For this review, take the finished solid that the model builds, in its own axes (mm). A direction names the side the tool comes from. Round coordinates to 2 decimals unless told otherwise and drop trailing zeros. Order: outer loops, then holes, each group sorted by start corner. A loop starts at its lowest first (then second) coordinate and runs counter-clockwise, first axis right, second up. Notation, with made-up numbers: (41.5, 38) -> (97.5, 38) arc R20 cw to (97.5, 54) -> close; hole circle Ø10 at (33.5, 9). An arc over 180 degrees is marked (long way). Use a Markdown table: item, result. Add a question column.
1) Machinability: for faces 1 (the face through (0.176, 5.803, -7.998)), 2 (the face through (6.05, 3, 6)), 3 (the face through (9.82, 2.96, 4.94)), which of the approach directions +Z, -Z, +X, -X, +Y, -Y give a long, thin tool a straight path to every point of the face, cutting with its end or side? Answer none if there is none.
2) Consider section C-C (y = 5.1). State the section outline as (x, z) points, plus the area to 3 significant figures.
3) Consider section A-A (x = 0). State the section outline as (y, z) points, plus the area to 3 significant figures.
4) Consider section B-B (z = -1.75). State the section outline as (x, y) points.
5) Consider section D-D (z = 9.5). State the section outline as (x, y) points.
6) Clearance check with flat-ended pins moving along their axes: P1, Ø1.7, axis at y = 2, z = 4.5, coming from the -X side; P2, Ø1.7, axis at y = 3.5, z = 6.5, coming from the +X side. State where each tip first meets the part, or that it passes through.
7) Wall thickness on line 1 along X through (y, z) = (0.9, 7.5); line 2 along X through (y, z) = (3.1, 7.25); line 3 along Z through (x, y) = (9.5, 1.45): over which ranges is each line inside the solid? List them lowest first. Write a range as [from, to].
8) Draft analysis for pull direction X (two halves, no side actions). For faces 4 (the face through (-0.58, 2.96, -17.96)), 5 (the face through (-10, 3, 11.795)), 6 (the face through (-6.05, 3, 6)), state which applies: pulls with the +X half, pulls with the -X half, needs draft (parallel to the pull), parting line crosses it, or undercut.
```python
from build123d import *

# Parameters (mm, degrees)
SKETCH1_R           = 1.65
SKETCH1_R_2         = 1
BOSS_EXTRUDE1_DEPTH = 6
CUT_EXTRUDE1_DEPTH  = 0.4


with BuildPart() as part:
    # Sketch1 → Boss-Extrude1 (new body)
    with BuildSketch(Plane(origin=(0, 0, 0), x_dir=(1, 0, 0), z_dir=(0, 1, 0))):
        with BuildLine():
            Line((13.55616119, -11.79495), (6.05, -11.79495))
            Line((6.05, -11.79495), (6.05, 0))
            ThreePointArc((6.05, 0), (0, 6.05), (-6.05, 0))
            Line((-6.05, 0), (-6.05, -11.79495))
            Line((-6.05, -11.79495), (-13.55616119, -11.79495))
            ThreePointArc((-13.55616119, -11.79495), (0, 17.96915), (13.55616119, -11.79495))
        make_face()
        with Locations(Location((-10.82295, 6.24955, 0), (0, 0, 270))):
            Circle(SKETCH1_R, mode=Mode.SUBTRACT)
        with Locations(Location((10.82295, 6.24955, 0), (0, 0, 270))):
            Circle(SKETCH1_R, mode=Mode.SUBTRACT)
        with Locations(Location((10.82295, -6.24955, 0), (0, 0, 270))):
            Circle(SKETCH1_R, mode=Mode.SUBTRACT)
        with Locations(Location((-10.82295, -6.24955, 0), (0, 0, 270))):
            Circle(SKETCH1_R, mode=Mode.SUBTRACT)
        with Locations(Location((0, 12.4985, 0), (0, 0, 270))):
            Circle(SKETCH1_R_2, mode=Mode.SUBTRACT)
    extrude(amount=BOSS_EXTRUDE1_DEPTH)

    # Sketch2 → Cut-Extrude1 (cut)
    with BuildSketch(Plane(origin=(0, 6, 0), x_dir=(1, 0, 0), z_dir=(0, 1, 0))):
        with BuildLine():
            Line((-8, 0), (-8, -11.79495))
            Line((-8, -11.79495), (8, -11.79495))
            Line((8, -11.79495), (8, 0))
            ThreePointArc((8, 0), (0, 8), (-8, 0))
        make_face()
    extrude(amount=-CUT_EXTRUDE1_DEPTH, mode=Mode.SUBTRACT)


solid = part.part
```
Results list:
| question | item | result |
|---|---|---|
| 1 | face 1 | +Z, +Y |
| 1 | face 2 | +Z, +Y, -Y |
| 1 | face 3 | +Y, -Y |
| 2 | outline | (-13.56, 11.79) arc R17.97 ccw (long way) to (13.56, 11.79) -> (6.05, 11.79) -> (6.05, 0) arc R6.05 cw to (-6.05, 0) -> (-6.05, 11.79) -> close; hole circle Ø3.3 at (-10.82, -6.25); hole circle Ø3.3 at (-10.82, 6.25); hole circle Ø2 at (0, -12.5); hole circle Ø3.3 at (10.82, -6.25); hole circle Ø3.3 at (10.82, 6.25) |
| 2 | area | 661 mm2 |
| 3 | outline | (0, -17.97) -> (6, -17.97) -> (6, -13.5) -> (0, -13.5) -> close; (0, -11.5) -> (6, -11.5) -> (6, -8) -> (5.6, -8) -> (5.6, -6.05) -> (0, -6.05) -> close |
| 3 | area | 58.7 mm2 |
| 4 | outline | (-17.88, 0) -> (-5.79, 0) -> (-5.79, 5.6) -> (-7.81, 5.6) -> (-7.81, 6) -> (-17.88, 6) -> close; (5.79, 0) -> (17.88, 0) -> (17.88, 6) -> (7.81, 6) -> (7.81, 5.6) -> (5.79, 5.6) -> close |
| 5 | outline | (-15.25, 0) -> (-6.05, 0) -> (-6.05, 5.6) -> (-8, 5.6) -> (-8, 6) -> (-15.25, 6) -> close; (6.05, 0) -> (15.25, 0) -> (15.25, 6) -> (8, 6) -> (8, 5.6) -> (6.05, 5.6) -> close |
| 6 | P1 | x = -17.59 |
| 6 | P2 | x = 17.06 |
| 7 | line 1 | [-16.33, -11.9], [-9.75, -6.05], [6.05, 9.75], [11.9, 16.33] |
| 7 | line 2 | [-16.44, -12.14], [-9.51, -6.05], [6.05, 9.51], [12.14, 16.44] |
| 7 | line 3 | [-15.25, -7.24], [-5.26, 5.26], [7.24, 11.79] |
| 8 | face 4 | parting line crosses it |
| 8 | face 5 | needs draft |
| 8 | face 6 | undercut |
